Check sheet for the modelled part. Datum: model origin and axes. Units: mm. Face numbers are marked on the shaded views. Coordinates: 2 decimals unless noted, no trailing zeros. Loops run counter-clockwise (first coordinate to the right, second up) from the corner with the lowest first, then second, coordinate; pieces in that order, holes last. Notation, with made-up numbers: (49, -26.5) - (63, -26.5) arc R16 cw to (63, -2.5) - close; hole circle Ø8 at (42.5, 44.5). An arc over 180 degrees is marked (long way). Use a Markdown table: item, result. Add a question column.
1) Thickness scan on line 1 (X direction, y = -22.5, z = 0.25); line 2 (Z direction, x = 0, y = -21.5); line 3 (Z direction, x = -3.75, y = -23.5). Record the ranges inside material, lowest first.
2) Go/stop test with flat-tipped pins: P1, Ø3, axis at x = 6, y = -31.5, coming from the +Z side; P2, Ø3, axis at y = -43, z = 2, coming from the -X side. Record where each tip stops, or that it passes through.
3) Draft check along X on the marked faces 1, 2 and 3. Enter one of: pulls with the +X half, pulls with the -X half, needs draft (parallel to the pull), parting line crosses it, or undercut.
4) Sectioned sample at A-A, the plane y = -13. Enter the section's corners in (x, z).
from build123d import *

# Parameters (mm, degrees)
F0_R     = 8
F1_DEPTH = 60
F3_D     = 8.5
F3_DEPTH = 35
F3_TIP   = 2.5536576309
F4_SIZE2 = 2.1159237685
F4_SIZE  = 12


with BuildPart() as f1:
    # F0 (on Front) → F1 (new body)
    with BuildSketch(Plane.XZ):
        Circle(F0_R)
    extrude(amount=F1_DEPTH)

    # F3
    with Locations(Plane(origin=(0, 0, 0), x_dir=(-1, 0, 0), z_dir=(0, 1, 0))):
        with Locations((0, 0)):
            Hole(F3_D / 2, depth=F3_DEPTH)
            with Locations((0, 0, -(F3_DEPTH + F3_TIP / 2))):  # 118° drill point
                Cone(0, F3_D / 2, F3_TIP, mode=Mode.SUBTRACT)

    # F4
    f4_edges = [f1.edges().sort_by_distance(p)[0] for p in [
        (-8, 0, 0),
    ]]
    f4_side = f1.faces().sort_by_distance((-8, -30, 0))[0]
    chamfer(f4_edges, length=F4_SIZE, length2=F4_SIZE2, reference=f4_side)


solid = f1.part
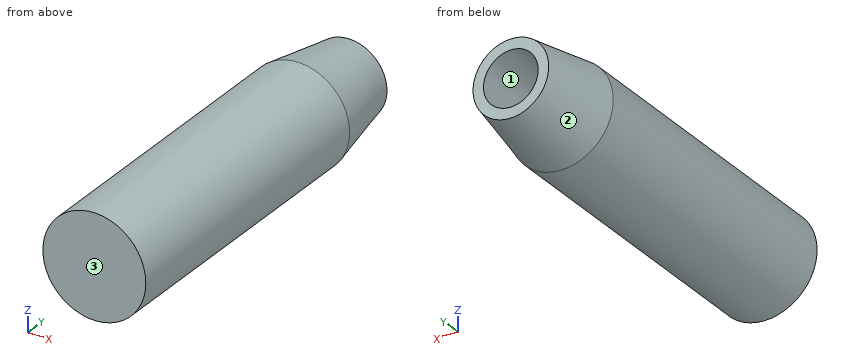
Solved:
| question | item | result |
|---|---|---|
| 1 | line 1 | x = -8 to -4.24, 4.24 to 8 |
| 1 | line 2 | z = -8 to -4.25, 4.25 to 8 |
| 1 | line 3 | z = -7.07 to -2, 2 to 7.07 |
| 2 | P1 | stops at z = 6.61 |
| 2 | P2 | stops at x = -7.98 |
| 3 | face 1 | undercut |
| 3 | face 2 | parting line crosses it |
| 3 | face 3 | needs draft |
| 4 | outline | circle Ø16 at (0, 0); hole circle Ø8.5 at (0, 0) |
